```python
from build123d import *

# Parameters (mm, degrees)
SKETCH_1_R          = 1.25
EXTRUDE_1_DEPTH     = 1.6
SKETCH_2_W          = 18
SKETCH_2_H          = 18
SKETCH_2_W_2        = 2.54
SKETCH_2_H_2        = 38.1
EXTRUDE_2_DEPTH     = 8
SKETCH_4_W          = 12.5
SKETCH_4_H          = 12.5
CUT_EXTRUDE_1_DEPTH = 5
SKETCH_5_W          = 0.6
SKETCH_5_H          = 0.6
EXTRUDE_3_DEPTH     = 6
CHAMFER_1_SIZE      = 0.5


with BuildPart() as part:
    # 草图1 → 凸台-拉伸1 (new body)
    with BuildSketch(Plane(origin=(0, 0, 0), x_dir=(1, 0, 0), z_dir=(0, 1, 0))):
        with BuildLine():
            Line((-10.25, -24.25), (10.25, -24.25))
            ThreePointArc((10.25, -24.25), (11.664213562, -23.664213562), (12.25, -22.25))
            Line((12.25, -22.25), (12.25, 22.25))
            ThreePointArc((12.25, 22.25), (11.664213562, 23.664213562), (10.25, 24.25))
            Line((10.25, 24.25), (-10.25, 24.25))
            ThreePointArc((-10.25, 24.25), (-11.664213562, 23.664213562), (-12.25, 22.25))
            Line((-12.25, 22.25), (-12.25, -22.25))
            ThreePointArc((-12.25, -22.25), (-11.664213562, -23.664213562), (-10.25, -24.25))
        make_face()
        with Locations(Location((-10.25, 22.25, 0), (0, 0, 270))):
            Circle(SKETCH_1_R, mode=Mode.SUBTRACT)
        with Locations(Location((10.25, 22.25, 0), (0, 0, 270))):
            Circle(SKETCH_1_R, mode=Mode.SUBTRACT)
        with Locations(Location((-10.25, -22.25, 0), (0, 0, 270))):
            Circle(SKETCH_1_R, mode=Mode.SUBTRACT)
        with Locations(Location((10.25, -22.25, 0), (0, 0, 270))):
            Circle(SKETCH_1_R, mode=Mode.SUBTRACT)
    extrude(amount=EXTRUDE_1_DEPTH)

    # 草图2 → 凸台-拉伸2 (add)
    with BuildSketch(Plane(origin=(0, 1.6, 0), x_dir=(1, 0, 0), z_dir=(0, 1, 0))):
        with Locations((0, 7.25)):
            Rectangle(SKETCH_2_W, SKETCH_2_H)
        with Locations((-10.98, 0)):
            Rectangle(SKETCH_2_W_2, SKETCH_2_H_2)
        with Locations((10.98, 0)):
            Rectangle(SKETCH_2_W_2, SKETCH_2_H_2)
    extrude(amount=EXTRUDE_2_DEPTH)

    # 草图4 → 切除-拉伸1 (cut)
    with BuildSketch(Plane(origin=(0, 9.6, 0), x_dir=(1, 0, 0), z_dir=(0, 1, 0))):
        with Locations((0, 7.25)):
            Rectangle(SKETCH_4_W, SKETCH_4_H)
    extrude(amount=-CUT_EXTRUDE_1_DEPTH, mode=Mode.SUBTRACT)

    # 草图5 → 凸台-拉伸3 (add)
    with BuildSketch(Plane(origin=(0, 9.6, 0), x_dir=(1, 0, 0), z_dir=(0, 1, 0))):
        with Locations((-10.98, 17.78)):
            Rectangle(SKETCH_5_W, SKETCH_5_H)
        with Locations((-10.98, 15.24)):
            Rectangle(SKETCH_5_W, SKETCH_5_H)
        with Locations((-10.98, 12.7)):
            Rectangle(SKETCH_5_W, SKETCH_5_H)
        with Locations((-10.98, 10.16)):
            Rectangle(SKETCH_5_W, SKETCH_5_H)
        with Locations((-10.98, 7.62)):
            Rectangle(SKETCH_5_W, SKETCH_5_H)
        with Locations((-10.98, 5.08)):
            Rectangle(SKETCH_5_W, SKETCH_5_H)
        with Locations((-10.98, 2.54)):
            Rectangle(SKETCH_5_W, SKETCH_5_H)
        with Locations((-10.98, 0)):
            Rectangle(SKETCH_5_W, SKETCH_5_H)
        with Locations((-10.98, -2.54)):
            Rectangle(SKETCH_5_W, SKETCH_5_H)
        with Locations((-10.98, -5.08)):
            Rectangle(SKETCH_5_W, SKETCH_5_H)
        with Locations((-10.98, -7.62)):
            Rectangle(SKETCH_5_W, SKETCH_5_H)
        with Locations((-10.98, -10.16)):
            Rectangle(SKETCH_5_W, SKETCH_5_H)
        with Locations((-10.98, -12.7)):
            Rectangle(SKETCH_5_W, SKETCH_5_H)
        with Locations((-10.98, -15.24)):
            Rectangle(SKETCH_5_W, SKETCH_5_H)
        with Locations((-10.98, -17.78)):
            Rectangle(SKETCH_5_W, SKETCH_5_H)
        with Locations((10.98, -17.78)):
            Rectangle(SKETCH_5_W, SKETCH_5_H)
        with Locations((10.98, -15.24)):
            Rectangle(SKETCH_5_W, SKETCH_5_H)
        with Locations((10.98, -12.7)):
            Rectangle(SKETCH_5_W, SKETCH_5_H)
        with Locations((10.98, -10.16)):
            Rectangle(SKETCH_5_W, SKETCH_5_H)
        with Locations((10.98, -7.62)):
            Rectangle(SKETCH_5_W, SKETCH_5_H)
        with Locations((10.98, -5.08)):
            Rectangle(SKETCH_5_W, SKETCH_5_H)
        with Locations((10.98, -2.54)):
            Rectangle(SKETCH_5_W, SKETCH_5_H)
        with Locations((10.98, 0)):
            Rectangle(SKETCH_5_W, SKETCH_5_H)
        with Locations((10.98, 2.54)):
            Rectangle(SKETCH_5_W, SKETCH_5_H)
        with Locations((10.98, 5.08)):
            Rectangle(SKETCH_5_W, SKETCH_5_H)
        with Locations((10.98, 7.62)):
            Rectangle(SKETCH_5_W, SKETCH_5_H)
        with Locations((10.98, 10.16)):
            Rectangle(SKETCH_5_W, SKETCH_5_H)
        with Locations((10.98, 12.7)):
            Rectangle(SKETCH_5_W, SKETCH_5_H)
        with Locations((10.98, 15.24)):
            Rectangle(SKETCH_5_W, SKETCH_5_H)
        with Locations((10.98, 17.78)):
            Rectangle(SKETCH_5_W, SKETCH_5_H)
    extrude(amount=EXTRUDE_3_DEPTH)

    # 倒角1
    chamfer_1_edges = [part.edges().sort_by_distance(p)[0] for p in [
        (9, 5.6, 1.75),
        (9, 5.6, -16.25),
        (-9, 5.6, -16.25),
        (-9, 5.6, 1.75),
        (-12.25, 5.6, -19.05),
        (-12.25, 5.6, 19.05),
        (-9.71, 5.6, 19.05),
        (-9.71, 5.6, -19.05),
        (12.25, 5.6, -19.05),
        (9.71, 5.6, -19.05),
        (9.71, 5.6, 19.05),
        (12.25, 5.6, 19.05),
        (6.25, 7.1, -13.5),
        (6.25, 7.1, -1),
        (-6.25, 7.1, -1),
        (-6.25, 7.1, -13.5),
    ]]
    chamfer(chamfer_1_edges, length=CHAMFER_1_SIZE)


solid = part.part
```
Could you check a few things on this model? Use its own coordinates, in mm. A direction names the side the tool comes from. Round coordinates to 2 decimals unless told otherwise and drop trailing zeros. Loops run counter-clockwise (first coordinate to the right, second up) from the corner with the lowest first, then second, coordinate; pieces in that order, holes last.
Q1. Please list where these lines run through material, in increasing order: L1, parallel to X at y = 0.8, z = 22.25; L2, parallel to Z at x = 2.5, y = 7.75; L3, parallel to Z at x = -10, y = 1.
Q2. I want a section at B-B (x = 3.5). Write out the boundary of the cut face in (y, z), and give its area (3 significant figures).
Q3. Thinking about a two-plate mould opening in X: for faces 6 (the flat face through (0, 1, 24.25)), 7 (the cylindrical face through (11.68, 0.79, -23.65)), 8 (the flat face through (-8, 9.6, -7)), 9 (the flat face through (-12.25, 5, 0)), which applies, pulls with the +X half, pulls with the -X half, needs draft (parallel to the pull), parting line crosses it, or undercut?
Q4. For P1, Ø2, axis at x = 4, z = 11.5, coming from the +Y side; P2, Ø1.5, axis at x = 8.5, y = 3, coming from the +Z side; P3, Ø0.7, axis at x = -11, y = 13, coming from the -Z side, each with a flat end and sliding along its axis, tell me the tip position at first contact or that it passes through.
Q5. On a 3-axis mill with a long thin cutter (end or side, diameter ignored), from which of +Z, -Z, +X, -X, +Y, -Y can I reach the whole of each face in a straight line? I mean faces 1 (the flat face through (-9.71, 6, 0)), 2 (the cylindrical face through (-9.87, 0.79, -21.06)), 3 (the flat face through (0, 6, -16.25)), 4 (the flat face through (6.25, 7, -7)), 5 (the flat face through (11, 6, 19.05)). Say none if no direction works.
Q6. I want a section at C-C (z = 4). Write out the boundary of the cut face in (x, y), and give its area (3 significant figures).
Q7. I want a section at A-A (y = 8). Give the number of separate pieces and of enclosed holes in the cut face, and give its area (3 significant figures).
Answer below:
1. L1: x = -12.25 to -11.5, -9 to 9, 11.5 to 12.25
1. L2: z = -16.25 to -13.5, -1 to 1.75
1. L3: z = -24.25 to -23.47, -21.03 to 21.03, 23.47 to 24.25
2. outline: (0, -24.25) - (1.6, -24.25) - (1.6, -16.25) - (9.6, -16.25) - (9.6, -13.5) - (4.6, -13.5) - (4.6, -1) - (9.6, -1) - (9.6, 1.75) - (1.6, 1.75) - (1.6, 24.25) - (0, 24.25) - close
2. area: 159 mm2
3. face 6: needs draft
3. face 7: pulls with the +X half
3. face 8: undercut
3. face 9: pulls with the -X half
4. P1: stops at y = 1.6
4. P2: stops at z = 1.75
4. P3: stops at z = -18.08
5. face 1: +Z, -Z, +Y
5. face 2: +Y, -Y
5. face 3: -Z, +Y
5. face 4: +Y
5. face 5: +Z, +X, -X, +Y
6. outline: (-12.25, 0) - (12.25, 0) - (12.25, 9.6) - (9.71, 9.6) - (9.71, 1.6) - (-9.71, 1.6) - (-9.71, 9.6) - (-12.25, 9.6) - close
6. area: 79.8 mm2
7. separate pieces: 3
7. enclosed holes: 1
7. area: 360 mm2
